from build123d import *

# Parameters (mm, degrees)
F1_DEPTH = 63.5
F2_DEPTH = 25.4
F3_DEPTH = 7.9375
F0_W     = 25.4
F0_H     = 28.575
F5_R     = 6.35


with BuildPart() as f1:
    # F0 (on Front) → F1 (new body, symmetric)
    with BuildSketch(Plane.XZ):
        Polygon((22.225, 9.525), (-41.275, 9.525), (-41.275, -9.525), (41.275, -9.525), (41.275, 9.525), align=None)
    extrude(amount=F1_DEPTH, both=True)

    # F0 (on Front) → F2 (join, symmetric)
    with BuildSketch(Plane.XZ):
        with BuildLine():
            Line((22.225, 27.0002), (22.225, 9.525))
            Line((22.225, 9.525), (41.275, 9.525))
            Line((41.275, 9.525), (41.275, 27.0002))
            ThreePointArc((41.275, 27.0002), (45.92468, 38.22552), (57.15, 42.8752))
            Line((57.15, 42.8752), (70.502212, 42.8752))
            Line((70.502212, 42.8752), (70.502212, 61.9252))
            Line((70.502212, 61.9252), (57.15, 61.9252))
            ThreePointArc((57.15, 61.9252), (32.454296, 51.695904), (22.225, 27.0002))
        make_face()
        Polygon((70.502212, 66.675), (70.502212, 61.9252), (70.502212, 42.8752), (70.502212, 38.1), (95.902212, 38.1), (95.902212, 66.675), align=None)
    extrude(amount=F2_DEPTH, both=True)

    # F0 (on Front) → F3 (join, symmetric)
    with BuildSketch(Plane.XZ):
        with BuildLine():
            add(Edge.make_bspline(
                [(-41.275, 9.525), (-36.434188, 37.679806), (-16.919576, 66.744119), (57.15, 61.9252)],
                knots=[0, 0, 0, 0, 111.504536, 111.504536, 111.504536, 111.504536], degree=3))
            Line((-41.275, 9.525), (22.225, 9.525))
            Line((22.225, 9.525), (22.225, 27.0002))
            ThreePointArc((22.225, 27.0002), (32.454296, 51.695904), (57.15, 61.9252))
        make_face()
    extrude(amount=F3_DEPTH, both=True)

    # F0 (on Front) → F4 (revolve)
    with BuildSketch(Plane.XZ):
        with Locations((108.602212, 52.3875)):
            Rectangle(F0_W, F0_H)
    revolve(axis=Axis((95.902212, 0, 52.3875), (0, 0, 1)))

    # F5
    f5_edges = [f1.edges().sort_by_distance(p)[0] for p in [
        (41.275, -63.5, 0),
        (-41.275, -63.5, 0),
        (41.275, 63.5, 0),
        (-41.275, 63.5, 0),
    ]]
    fillet(f5_edges, radius=F5_R)


solid = f1.part
CAD build for the part. Positions are in the model's coordinates, mm. A direction names the side the tool comes from. Round coordinates to 2 decimals unless told otherwise and drop trailing zeros. Write each loop counter-clockwise with the first axis right and the second up, starting at its lowest first coordinate (ties: lowest second). Pieces come first, ordered by that corner, then holes. Notation, with made-up numbers: M 77.25,-15.75 L 126.25,-15.75 A20 ccw 126.25,8.25 Z; hole C 13,-3 d9. An arc over 180 degrees is marked long. Put each result on its own line as item: value. Start each with the question number.
1) Saw through at C-C, the plane y = -16. Write the cut outline in (x, z) (3 decimals).
2) Pull direction X, two halves, no side cores. Call faces 4 (the flat face through (96, 0, 66.675)), 5 (the cylindrical face through (32.73, -16.79, 51.97)), 6 (the cylindrical face through (45.8, -0.4, 38.1)): pulls with the +X half, pulls with the -X half, needs draft (parallel to the pull), parting line crosses it, or undercut.
3) Drill centre lines: probe 1 along Z at (x, y) = (25, -45) (3 decimals); probe 2 along Y at (x, z) = (17.5, 29); probe 3 along Z at (x, y) = (57.5, 1). Where is each one in solid material? Low to high. Write a range as [from, to].
4) 3-axis set-ups, long thin cutter, end or side, ignore diameter. For faces 1 (the flat face through (96, 0, 38.1)), 2 (the flat face through (64, 0, 61.925)), 3 (the flat face through (64, 0, 42.875)): which of +Z, -Z, +X, -X, +Y, -Y reach the whole face in a straight line?
5) Saw through at B-B, the plane y = 12. Write the cut outline in (x, z) (3 decimals).
6) Saw through at D-D, the plane y = 45. Write the cut outline in (x, z) (3 decimals), and give its area (3 significant figures).
7) Pin check, flat tips, straight feed: pin 1 Ø5 at (y, z) = (21, 20) entering from -X (3 decimals); pin 2 Ø12 at (x, z) = (-9, 34.5) entering from +Y; pin 3 Ø3 at (y, z) = (-12.5, 11) entering from +X (3 decimals). Stop position of each tip, or through.
8) Saw through at A-A, the plane z = 3. Write the cut outline in (x, y) (3 decimals), and give its area (3 significant figures).
Resolved:
1. outline: M -41.275,-9.525 L 41.275,-9.525 L 41.275,27 A15.875 cw 57.15,42.875 L 70.502,42.875 L 70.502,38.1 L 115.629,38.1 L 115.629,66.675 L 70.502,66.675 L 70.502,61.925 L 57.15,61.925 A34.925 ccw 22.225,27 L 22.225,9.525 L -41.275,9.525 Z
2. face 4: needs draft
2. face 5: pulls with the -X half
2. face 6: undercut
3. probe 1: [-9.525, 9.525]
3. probe 2: [-7.94, 7.94]
3. probe 3: [42.88, 61.93]
4. face 1: -Z, +X, +Y, -Y
4. face 2: +Z, +Y, -Y
4. face 3: -Z, +Y, -Y
5. outline: M -41.275,-9.525 L 41.275,-9.525 L 41.275,27 A15.875 cw 57.15,42.875 L 70.502,42.875 L 70.502,38.1 L 118.289,38.1 L 118.289,66.675 L 70.502,66.675 L 70.502,61.925 L 57.15,61.925 A34.925 ccw 22.225,27 L 22.225,9.525 L -41.275,9.525 Z
6. outline: M -41.275,-9.525 L 41.275,-9.525 L 41.275,9.525 L -41.275,9.525 Z
6. area: 1,570 mm²
7. pin 1: x = 22.225
7. pin 2: y = 7.94
7. pin 3: x = 41.275
8. outline: M -41.275,-57.15 A6.35 ccw -34.925,-63.5 L 34.925,-63.5 A6.35 ccw 41.275,-57.15 L 41.275,57.15 A6.35 ccw 34.925,63.5 L -34.925,63.5 A6.35 ccw -41.275,57.15 Z
8. area: 10,400 mm²
